The model under review builds one solid part; all positions refer to its coordinate system, in mm. A direction names the side the tool comes from. Coordinates: 2 decimals unless noted, no trailing zeros. Write each loop counter-clockwise with the first axis right and the second up, starting at its lowest first coordinate (ties: lowest second). Pieces come first, ordered by that corner, then holes. Notation, with made-up numbers: M 3.25,48 L 8.25,48 A22 ccw 8.25,71 Z; hole C 19.25,69.5 d2. An arc over 180 degrees is marked long. Answer as CSV lines item,"result". Start each with the question number.
from build123d import *

# Parameters (mm, degrees)
SKETCH1_R           = 1.5
BOSS_EXTRUDE1_DEPTH = 2.7
FILLET1_R           = 0.15
FILLET2_R           = 1
FILLET3_R           = 1
FILLET4_R           = 1
SCALE1_SCALE        = 1.9


with BuildPart() as part:
    # Sketch1 → Boss-Extrude1 (new body)
    with BuildSketch(Plane.XY):
        with BuildLine():
            Line((0, 5), (19.85, 5))
            Line((19.85, 5), (45.99619398, 15.75))
            Line((45.99619398, 15.75), (52.557536486, 12.761206845))
            Line((52.557536486, 12.761206845), (53.907471601, 9.477889135))
            ThreePointArc((53.907471601, 9.477889135), (53.977314115, 8.995006796), (53.810360044, 8.536553233))
            Line((53.810360044, 8.536553233), (53.148294507, 7.559788561))
            Line((53.148294507, 7.559788561), (52.056234711, 8.006784537))
            Line((52.056234711, 8.006784537), (51.394169174, 7.030019865))
            Line((51.394169174, 7.030019865), (50.302109378, 7.477015841))
            Line((50.302109378, 7.477015841), (49.640043841, 6.500251169))
            Line((49.640043841, 6.500251169), (48.547984045, 6.947247144))
            Line((48.547984045, 6.947247144), (47.885918508, 5.970482472))
            Line((47.885918508, 5.970482472), (46.793858712, 6.417478448))
            Line((46.793858712, 6.417478448), (46.131793175, 5.440713776))
            ThreePointArc((46.131793175, 5.440713776), (46.03170075, 5.315863389), (45.912975416, 5.208576821))
            Line((45.912975416, 5.208576821), (44.507662892, 4.129714813))
            ThreePointArc((44.507662892, 4.129714813), (44.031433487, 3.93177062), (43.519903831, 3.997449854))
            Line((43.519903831, 3.997449854), (38.212047423, 6.170032768))
            Line((38.212047423, 6.170032768), (25.644379319, 1.158584034))
            Line((25.644379319, 1.158584034), (21.47, -5))
            Line((21.47, -5), (0, -5))
            ThreePointArc((0, -5), (-5, 0), (0, 5))
        make_face()
        Circle(SKETCH1_R, mode=Mode.SUBTRACT)
        with Locations((22, 0)):
            Circle(SKETCH1_R, mode=Mode.SUBTRACT)
    extrude(amount=-BOSS_EXTRUDE1_DEPTH)

    # Fillet1
    fillet1_edges = [part.edges().sort_by_distance(p)[0] for p in [
        (53.148294507, 7.559788561, -1.35),
        (51.394169174, 7.030019865, -1.35),
        (49.640043841, 6.500251169, -1.35),
        (47.885918508, 5.970482472, -1.35),
    ]]
    fillet(fillet1_edges, radius=FILLET1_R)

    # Fillet2
    fillet2_edges = [part.edges().sort_by_distance(p)[0] for p in [
        (21.47, -5, -1.35),
        (45.99619398, 15.75, -1.35),
        (52.557536486, 12.761206845, -1.35),
    ]]
    fillet(fillet2_edges, radius=FILLET2_R)

    # Fillet3
    fillet3_edges = [part.edges().sort_by_distance(p)[0] for p in [
        (38.212047423, 6.170032768, -1.35),
        (25.644379319, 1.158584034, -1.35),
    ]]
    fillet(fillet3_edges, radius=FILLET3_R)

    # Fillet4
    fillet4_edges = [part.edges().sort_by_distance(p)[0] for p in [
        (19.85, 5, -1.35),
    ]]
    fillet(fillet4_edges, radius=FILLET4_R)


with BuildPart() as part_1:
    # Scale1: scaled about (23.156973948, 3.883277681, -1.35)
    add(part.part.scale(SCALE1_SCALE).moved(Location((-20.841276553, -3.494949913, 1.215))))


solid = part_1.part
1) Clearance check with flat-ended pins moving along their axes: pin 1 Ø3 at (x, z) = (59.5, 0.5) entering from +Y; pin 2 Ø3 at (y, z) = (19.5, 0.5) entering from -X; pin 3 Ø2.5 at (x, z) = (4.5, -2) entering from +Y; pin 4 Ø3.5 at (x, y) = (-20.84, -3.49) entering from -Z. State where each tip first meets the part, or that it passes through.
2) Tool access review of faces 1 (the flat face through (-2, 6.005, -1)), 2 (the flat face through (65.077, 5.391, -1.314)), 3 (the flat face through (39.9, 3.5, -1.3)): name each direction out of +Z, -Z, +X, -X, +Y, -Y from which nothing blocks a thin tool from reaching the whole face with its end or side.
3) Take a section at B-B on y = 23. Give the boundary of the cut face in (x, z) (3 decimals), and give its area (3 significant figures).
4) Take a section at A-A on z = -2.25. Give the number of separate pieces and of enclosed holes in the cut face, and give its area (3 significant figures).
5) Take a section at C-C on x = 59. Give the boundary of the cut face in (y, z) (3 decimals).
6) To check wall thickness, follow line 1 (X direction, y = -4, z = -2.8); line 2 (Y direction, x = 22, z = 0.15); line 3 (Y direction, x = 0.5, z = -3.6). State the ranges of each line that lie inside material, in increasing order. Write a range as [from, to].
Results:
1,pin 1,"stops at y = 24.15"
1,pin 2,"stops at x = 46.05"
1,pin 3,"stops at y = 6.01"
1,pin 4,"passes through"
2,face 1,"+Z, -Z, -X, +Y"
2,face 2,"+Z, -Z, +X, -Y"
2,face 3,"+Z, -Z, -Y"
3,outline,"M 58.209,-3.915 L 74.082,-3.915 L 74.082,1.215 L 58.209,1.215 Z"
3,area,"81.4 mm²"
4,separate pieces,"1"
4,enclosed holes,"2"
4,area,"1,730 mm²"
5,outline,"M 5.265,-3.915 L 23.325,-3.915 L 23.325,1.215 L 5.265,1.215 Z"
6,line 1,"x = [-30.33, -23.65], [-18.04, 18.15], [23.76, 26.05]"
6,line 2,"y = [-9.97, -6.15], [-0.84, 8.11]"
6,line 3,"y = [-12.99, 6.01]"
